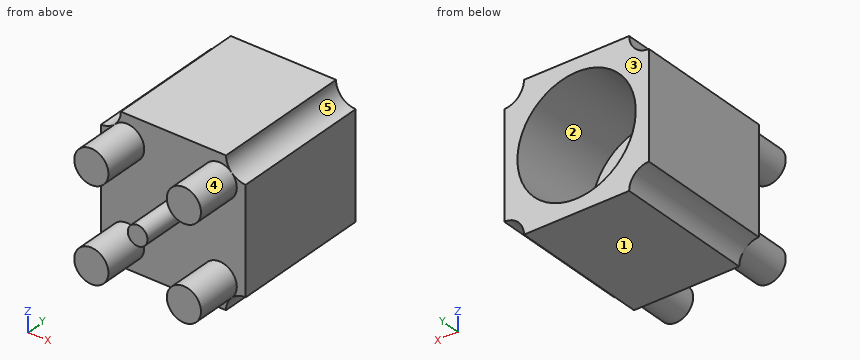
Autodesk Inventor part; units mm, degrees
ref_plane "YZ Plane" through (0, 0, 0) normal (1, 0, 0) x (0, 1, 0)
ref_plane "XZ Plane" through (0, 0, 0) normal (0, 1, 0) x (-1, 0, 0)
ref_plane "XY Plane" through (0, 0, 0) normal (0, 0, 1) x (1, 0, 0)
sketch "Sketch1" plane through (0, 0, 0) normal (0, 1, 0) x (-1, 0, 0)
  line L0 (-11, 11) -> (11, 11)
  line L1 (11, 11) -> (11, -11)
  line L2 (11, -11) -> (-11, -11)
  line L3 (-11, -11) -> (-11, 11)
  line L4 (-11, 11) -> (11, -11) construction
  line L5 (11, 11) -> (-11, -11) construction
  point P0 (0, 0)
  dimension "d0" = 22
  dimension "d1" = 22
extrude "Extrusion1" add sketch "Sketch1" along normal blind 28.5
sketch "Sketch2" plane through (0, 28.5, 0) normal (0, 1, 0) x (1, 0, 0)
  circle A0 centre (0, 0) radius 9
  dimension "d4" = 18
extrude "Extrusion2" cut sketch "Sketch2" against normal blind 14.5
sketch "Sketch3" plane through (0, 0, 0) normal (0, -1, 0) x (1, 0, 0)
  line L0 (11, 11) -> (-11, 11)
  line L1 (-11, 11) -> (-11, -11)
  line L2 (-11, -11) -> (11, -11)
  line L3 (11, -11) -> (11, 11)
  line L4 (11, 11) -> (11, -11)
  circle A0 centre (11, -11) radius 3
  line L5 (11, -11) -> (-11, -11)
  circle A1 centre (-11, -11) radius 3
  line L6 (-11, 11) -> (11, 11)
  circle A2 centre (-11, 11) radius 3
  circle A3 centre (11, 11) radius 3
  point P0 (0, 0)
  dimension "d7" = 6
  dimension "d8" = 6
  dimension "d9" = 6
  dimension "d10" = 6
extrude "Extrusion3" cut sketch "Sketch3" against normal through all contours A2 L1 L0 | L0 L1 A2 | A3 L3 L0 | L0 L3 A3 | A1 L2 L1 | L1 L2 A1 | A0 L2 L3 | L3 L2 A0
sketch "Sketch4" plane through (0, 0, 0) normal (0, -1, 0) x (1, 0, 0)
  circle A0 centre (0, 0) radius 1.5
  arc A1 (8, 11) -> (11, 8) centre (11, 11) ccw
  line L0 (8, 11) -> (-8, 11)
  arc A2 (-11, 8) -> (-8, 11) centre (-11, 11) ccw
  line L1 (-11, 8) -> (-11, -8)
  arc A3 (-8, -11) -> (-11, -8) centre (-11, -11) ccw
  line L2 (-8, -11) -> (8, -11)
  arc A4 (11, -8) -> (8, -11) centre (11, -11) ccw
  line L3 (11, -8) -> (11, 8)
  line L4 (7.0402, 7.0402) -> (4.4402, 7.0402)
  line L5 (-7.0402, 7.0402) -> (-7.0402, 4.4402)
  line L6 (-7.0402, -7.0402) -> (-4.4402, -7.0402)
  line L7 (7.0402, -7.0402) -> (7.0402, -4.4402)
  line L8 (7.0402, 7.0402) -> (-7.0402, -7.0402) construction
  line L9 (-7.0402, 7.0402) -> (7.0402, -7.0402) construction
  circle A5 centre (-7.0402, -7.0402) radius 2.6
  circle A6 centre (-7.0402, 7.0402) radius 2.6
  circle A7 centre (7.0402, 7.0402) radius 2.6
  circle A8 centre (7.0402, -7.0402) radius 2.6
  line L10 (-4.4402, -7.0402) -> (4.4402, -7.0402)
  line L11 (-7.0402, 4.4402) -> (-7.0402, -4.4402)
  line L12 (-7.0402, -4.4402) -> (-7.0402, -7.0402)
  line L13 (4.4402, -7.0402) -> (7.0402, -7.0402)
  line L14 (7.0402, -4.4402) -> (7.0402, 4.4402)
  line L15 (7.0402, 4.4402) -> (7.0402, 7.0402)
  line L16 (4.4402, 7.0402) -> (-4.4402, 7.0402)
  line L17 (-4.4402, 7.0402) -> (-7.0402, 7.0402)
  dimension "d13" = 3
  dimension "d15" = 14.0804
  dimension "d16" = 5.2
  dimension "d17" = 5.2
  dimension "d18" = 5.2
  dimension "d19" = 5.2
  dimension "d20" = 14.0804
extrude "Extrusion4" cut sketch "Sketch4" against normal blind 7 contours A1 A7 L16 A6 A2 L0 | A1 L3 A4 A8 L14 A7 | A7 L14 A8 L10 A5 L11 A6 L16 | A6 L11 A5 A3 L1 A2 | A4 L2 A3 A5 L10 A8
equation "\"d1\" = d0"
equation "\"d15\" = d20"
equation "\"d17\" = d16"
equation "\"d18\" = d17"
equation "\"d19\" = d18"
properties part number "VRUZEND_Caps"
Read the model definition and answer for the solid it produces. Units are mm, in the model's axes. Face numbers are marked on the shaded views. A direction names the side the tool comes from. Coordinates: 2 decimals unless noted, no trailing zeros. Write each loop counter-clockwise with the first axis right and the second up, starting at its lowest first coordinate (ties: lowest second). Pieces come first, ordered by that corner, then holes. Notation, with made-up numbers: (64.5, 31) -> (117.5, 31) arc R30 cw to (117.5, 67) -> close; hole circle Ø9 at (-16.75, -14). An arc over 180 degrees is marked (long way). Return JSON: item names as keys, results as strings.
(1) Consider line 1 along X through (y, z) = (25.5, 0); line 2 along Y through (x, z) = (8.25, -2.5). Determine where each line is inside the solid, lowest interval first. Write a range as from..to.
Answers below:
{"line 1": "-11..-9, 9..11", "line 2": "7..14"}
(2) The part is cut by section C-C on x = 0. Give the vertices of the cut face in (y, z).
Answers below:
{"outline": "(0, -1.5) -> (7, -1.5) -> (7, -11) -> (28.5, -11) -> (28.5, -9) -> (14, -9) -> (14, 9) -> (28.5, 9) -> (28.5, 11) -> (7, 11) -> (7, 1.5) -> (0, 1.5) -> close"}
(3) Which of the six approach directions +Z, -Z, +X, -X, +Y, -Y give full straight-line access (tool end or side, diameter ignored) to the marked faces 4 and 5?
Answers below:
{"face 4": "-Y", "face 5": "+Z, +X, +Y, -Y"}
(4) For a pull along Z with two mould halves and no side action, classify the marked faces 1, 2 and 3 as pulls with the +Z half, pulls with the -Z half, needs draft (parallel to the pull), parting line crosses it, or undercut.
Answers below:
{"face 1": "pulls with the -Z half", "face 2": "undercut", "face 3": "needs draft"}
(5) This flat-tipped pin is pushed along its axis until it touches: P1, Ø4, axis at x = -8, z = -4, coming from the +Y side. Where does it stop, or does it pass through?
Answers below:
{"P1": "y = 28.5"}
(6) The part is cut by section A-A on y = 19.5. Give the vertices of the cut face in (x, z).
Answers below:
{"outline": "(-11, -8) arc R3 cw to (-8, -11) -> (8, -11) arc R3 cw to (11, -8) -> (11, 8) arc R3 cw to (8, 11) -> (-8, 11) arc R3 cw to (-11, 8) -> close; hole circle Ø18 at (0, 0)"}
(7) The part is cut by section B-B on z = 0. Give the vertices of the cut face in (x, y), then the cut area to 3 significant figures.
Answers below:
{"outline": "(-11, 7) -> (-1.5, 7) -> (-1.5, 0) -> (1.5, 0) -> (1.5, 7) -> (11, 7) -> (11, 28.5) -> (9, 28.5) -> (9, 14) -> (-9, 14) -> (-9, 28.5) -> (-11, 28.5) -> close", "area": "233 mm^2"}
(8) The part is cut by section D-D on y = 2. Give the vertices of the cut face in (x, z).
Answers below:
{"outline": "circle Ø5.2 at (-7.04, -7.04); circle Ø5.2 at (-7.04, 7.04); circle Ø3 at (0, 0); circle Ø5.2 at (7.04, -7.04); circle Ø5.2 at (7.04, 7.04)"}
